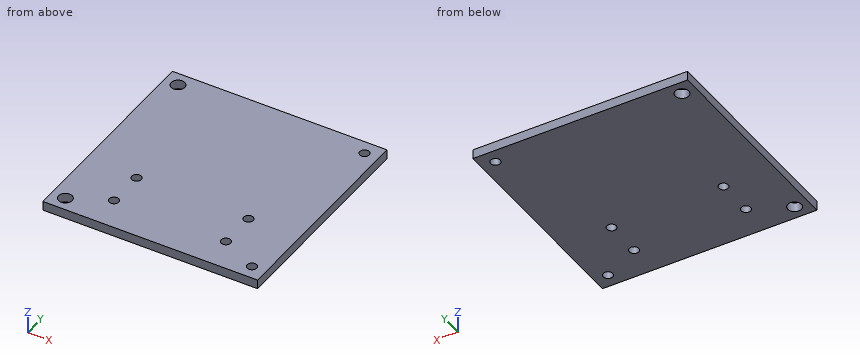
```python
from build123d import *

# Parameters (mm, degrees)
F1_W     = 115
F1_H     = 115
F1_W_2   = 100
F1_H_2   = 100
F2_DEPTH = 5
F3_D     = 5.1
F0_D     = 7.3
F5_D     = 5.1


with BuildPart() as f2:
    # F1 (on Top) → F2 (new body)
    with BuildSketch(Plane.XY):
        Rectangle(F1_W, F1_H)
        Rectangle(F1_W_2, F1_H_2, mode=Mode.SUBTRACT)
        Rectangle(F1_W_2, F1_H_2)
    extrude(amount=F2_DEPTH)

    # F3 (through all)
    with Locations(Plane(origin=(0, 0, 0), x_dir=(1, 0, 0), z_dir=(0, 0, -1))):
        with Locations((50, 50), (50, -50)):
            Hole(F3_D / 2)

    # F0 (through all)
    with Locations(Plane(origin=(0, 0, 0), x_dir=(1, 0, 0), z_dir=(0, 0, -1))):
        with Locations((-50, -50), (-50, 50)):
            Hole(F0_D / 2)

    # F5 (through all)
    with Locations(Plane.XY.offset(5)):
        with Locations((30, -20), (30, -40), (-30, -20), (-30, -40)):
            Hole(F5_D / 2)


solid = f2.part
```
Can you work these out from the model? Positions are in its coordinate system, mm. Coordinates: 2 decimals unless noted, no trailing zeros. Loops run counter-clockwise (first coordinate to the right, second up) from the corner with the lowest first, then second, coordinate; pieces in that order, holes last. Notation, with made-up numbers: M 55.5,-5.5 L 110.5,-5.5 A29 cw 110.5,18.5 Z; hole C 75.5,51.5 d1. An arc over 180 degrees is marked long. Put each result on its own line as item: value. Start each with the question number.
(1) Imagine slicing it at B-B on x = 50. List the corners of the cut face in (y, z) for me.
(2) I need wall thicknesses on probe 1 along X at (y, z) = (50, 1.45); probe 2 along Y at (x, z) = (30, 1.75); probe 3 along Y at (x, z) = (-50, 3.45). Which ranges of each line are inside material? Lowest first, please.
(3) Imagine slicing it at C-C on z = 3.45. Give the number of separate pieces and of enclosed holes in the cut face, and give its area (3 significant figures).
(4) Will these pins go through, and if not, where does the flat tip stop? pin 1 Ø4 at (x, y) = (30, -20) entering from -Z; pin 2 Ø6.5 at (x, y) = (-30, -20) entering from -Z.
(5) Imagine slicing it at A-A on y = -50. List the corners of the cut face in (x, z) for me.
Worked answers:
1. outline: M -57.5,0 L -52.55,0 L -52.55,5 L -57.5,5 Z; M -47.45,0 L 47.45,0 L 47.45,5 L -47.45,5 Z; M 52.55,0 L 57.5,0 L 57.5,5 L 52.55,5 Z
2. probe 1: x = -57.5 to -53.65, -46.35 to 47.45, 52.55 to 57.5
2. probe 2: y = -57.5 to -42.55, -37.45 to -22.55, -17.45 to 57.5
2. probe 3: y = -57.5 to -53.65, -46.35 to 46.35, 53.65 to 57.5
3. separate pieces: 1
3. enclosed holes: 8
3. area: 13,000 mm2
4. pin 1: passes through
4. pin 2: stops at z = 0
5. outline: M -57.5,0 L -53.65,0 L -53.65,5 L -57.5,5 Z; M -46.35,0 L 47.45,0 L 47.45,5 L -46.35,5 Z; M 52.55,0 L 57.5,0 L 57.5,5 L 52.55,5 Z
